Verification items for the finished model (mm, model axes). A direction names the side the tool comes from. Coordinates: 2 decimals unless noted, no trailing zeros. Write each loop counter-clockwise with the first axis right and the second up, starting at its lowest first coordinate (ties: lowest second). Pieces come first, ordered by that corner, then holes. Notation, with made-up numbers: (60.25, 72.25) -> (68.25, 72.25) arc R21 cw to (68.25, 95.25) -> close; hole circle Ø4 at (68.25, 62). An arc over 180 degrees is marked (long way). Answer in a Markdown table with one row per item.
```python
from build123d import *

# Parameters (mm, degrees)
SKETCH_1_W          = 12
SKETCH_1_H          = 12
EXTRUDE_1_DEPTH     = 15
SKETCH_2_W          = 6.4
SKETCH_2_H          = 12.2
CUT_EXTRUDE_1_DEPTH = 12
CUT_EXTRUDE_2_DEPTH = 12
SKETCH_8_R          = 2
CUT_EXTRUDE_3_DEPTH = 21.124611797
SKETCH_10_W         = 6
SKETCH_10_H         = 12
SKETCH_10_R         = 1.5
EXTRUDE_2_DEPTH     = 2.8


with BuildPart() as part:
    # 草图1 → 凸台-拉伸1 (new body)
    with BuildSketch(Plane(origin=(0, 0, 0), x_dir=(1, 0, 0), z_dir=(0, 1, 0))):
        Rectangle(SKETCH_1_W, SKETCH_1_H)
    extrude(amount=EXTRUDE_1_DEPTH)

    # 草图2 → 切除-拉伸1 (cut)
    with BuildSketch(Plane.XY.offset(6)):
        with Locations((0, 8.9)):
            Rectangle(SKETCH_2_W, SKETCH_2_H)
    extrude(amount=-CUT_EXTRUDE_1_DEPTH, mode=Mode.SUBTRACT)

    # 草图3 → 切除-拉伸2 (cut)
    with BuildSketch(Plane.ZY.offset(6)):
        with BuildLine():
            Line((-6, 15), (-6, 2.8))
            Line((-6, 2.8), (-1.658241819, 12.617796896))
            ThreePointArc((-1.658241819, 12.617796896), (-0.18275198, 14.351953728), (2, 15))
            Line((2, 15), (-6, 15))
        make_face()
        with BuildLine():
            ThreePointArc((2, 15), (4.828427125, 13.828427125), (6, 11))
            Line((6, 11), (6, 15))
            Line((6, 15), (2, 15))
        make_face()
    extrude(amount=-CUT_EXTRUDE_2_DEPTH, mode=Mode.SUBTRACT)

    # 草图8 → 切除-拉伸3 (cut, through all)
    with BuildSketch(Plane(origin=(6, 0, 0), x_dir=(0, 0, -1), z_dir=(1, 0, 0))):
        with Locations((-2, 11)):
            Circle(SKETCH_8_R)
    extrude(amount=-CUT_EXTRUDE_3_DEPTH, mode=Mode.SUBTRACT)

    # 草图10 → 凸台-拉伸2 (add)
    # profile 1 of 2: a face of its own
    with BuildSketch(Plane(origin=(0, 0, 0), x_dir=(1, 0, 0), z_dir=(0, 1, 0))):
        with Locations((-9, 0)):
            Rectangle(SKETCH_10_W, SKETCH_10_H)
        with Locations(Location((-9, 3, 0), (0, 0, 90))):
            Circle(SKETCH_10_R, mode=Mode.SUBTRACT)
        with Locations(Location((-9, -3, 0), (0, 0, 90))):
            Circle(SKETCH_10_R, mode=Mode.SUBTRACT)
    # profile 2 of 2: a face of its own
    with BuildSketch(Plane(origin=(0, 0, 0), x_dir=(1, 0, 0), z_dir=(0, 1, 0))):
        with Locations((9, 0)):
            Rectangle(SKETCH_10_W, SKETCH_10_H)
        with Locations(Location((9, 3, 0), (0, 0, 90))):
            Circle(SKETCH_10_R, mode=Mode.SUBTRACT)
        with Locations(Location((9, -3, 0), (0, 0, 90))):
            Circle(SKETCH_10_R, mode=Mode.SUBTRACT)
    extrude(amount=EXTRUDE_2_DEPTH)


solid = part.part
```
1. Tool access check on faces 1 (the flat face through (0, 2.8, 0)), 2 (the flat face through (-9, 2.8, 0)), 3 (the flat face through (0, 0, 0)). Record the directions out of +Z, -Z, +X, -X, +Y, -Y that give a thin tool (end or side, any length) a straight path to the whole face; none if there is none.
Geometry says:
| item | result |
|---|---|
| face 1 | +Z, -Z, +Y |
| face 2 | +Z, -Z, -X, +Y |
| face 3 | +Z, -Z, +X, -X, -Y |
2. Section check D-D, the plane x = 4. Record the boundary of the cut face in (y, z), plus the area to 3 significant figures.
Geometry says:
| item | result |
|---|---|
| outline | (0, -6) -> (2.8, -6) -> (12.62, -1.66) arc R4 ccw to (11, 6) -> (0, 6) -> close; hole circle Ø4 at (11, 2) |
| area | 130 mm^2 |
3. Section check B-B, the plane z = -2.5. Record the boundary of the cut face in (x, y).
Geometry says:
| item | result |
|---|---|
| outline | (-12, 0) -> (-10.41, 0) -> (-10.41, 2.8) -> (-12, 2.8) -> close; (-7.59, 0) -> (7.59, 0) -> (7.59, 2.8) -> (6, 2.8) -> (6, 10.71) -> (3.2, 10.71) -> (3.2, 2.8) -> (-3.2, 2.8) -> (-3.2, 10.71) -> (-6, 10.71) -> (-6, 2.8) -> (-7.59, 2.8) -> close; (10.41, 0) -> (12, 0) -> (12, 2.8) -> (10.41, 2.8) -> close |
4. Mould release check, pull along X, two halves, no side actions. Record for faces 4 (the flat face through (9, 2.8, 0)), 5 (the flat face through (6, 7, 1)), 6 (the flat face through (-3.2, 7, 1)): released by +X, released by -X, zero draft, split by the parting line, or undercut.
Geometry says:
| item | result |
|---|---|
| face 4 | zero draft |
| face 5 | released by +X |
| face 6 | undercut |
5. Section check A-A, the plane x = -9. Record the boundary of the cut face in (y, z), plus the area to 3 significant figures.
Geometry says:
| item | result |
|---|---|
| outline | (0, -6) -> (2.8, -6) -> (2.8, -4.5) -> (0, -4.5) -> close; (0, -1.5) -> (2.8, -1.5) -> (2.8, 1.5) -> (0, 1.5) -> close; (0, 4.5) -> (2.8, 4.5) -> (2.8, 6) -> (0, 6) -> close |
| area | 16.8 mm^2 |
6. Thickness scan on line 1 (Z direction, x = 9, y = 1.8); line 2 (X direction, y = 1.35, z = -3); line 3 (X direction, y = 6, z = 4.75). Record the ranges inside material, lowest first. Write a range as from..to.
Geometry says:
| item | result |
|---|---|
| line 1 | -6..-4.5, -1.5..1.5, 4.5..6 |
| line 2 | -12..-10.5, -7.5..7.5, 10.5..12 |
| line 3 | -6..-3.2, 3.2..6 |
7. Depth check by flat-ended pin: P1, Ø1.9, axis at x = 0.5, z = 3, coming from the +Y side; P2, Ø6, axis at x = 0.5, y = 6, coming from the +Z side; P3, Ø2, axis at y = 12.5, z = 4.5, coming from the -X side; P4, Ø6, axis at y = 11, z = -3, coming from the +X side. Enter the tip coordinate at first touch or a pass-through.
Geometry says:
| item | result |
|---|---|
| P1 | y = 2.8 |
| P2 | z = 6 |
| P3 | x = -6 |
| P4 | x = 6 |
8. Section check C-C, the plane y = 9.5. Record the boundary of the cut face in (x, z), plus the area to 3 significant figures.
Geometry says:
| item | result |
|---|---|
| outline | (-6, -3.04) -> (-3.2, -3.04) -> (-3.2, 0.68) -> (-6, 0.68) -> close; (-6, 3.32) -> (-3.2, 3.32) -> (-3.2, 6) -> (-6, 6) -> close; (3.2, -3.04) -> (6, -3.04) -> (6, 0.68) -> (3.2, 0.68) -> close; (3.2, 3.32) -> (6, 3.32) -> (6, 6) -> (3.2, 6) -> close |
| area | 35.8 mm^2 |
